from build123d import *

# Parameters (mm, degrees)
SKETCH1_W           = 77
SKETCH1_H           = 60
SKETCH1_W_2         = 71
SKETCH1_H_2         = 54
SKETCH1_R           = 1.75
BOSS_EXTRUDE1_DEPTH = 45
SKETCH2_R           = 1.75
CUT_EXTRUDE1_DEPTH  = 12
SKETCH3_W           = 77
SKETCH3_H           = 60
SKETCH3_R           = 1.75
BOSS_EXTRUDE2_DEPTH = 3
CUT_EXTRUDE2_DEPTH  = 10
SKETCH6_W           = 14
SKETCH6_H           = 9
CUT_EXTRUDE3_DEPTH  = 10
SKETCH7_R           = 1.1
CUT_EXTRUDE4_DEPTH  = 10
SKETCH9_W           = 60
SKETCH9_H           = 30
CUT_EXTRUDE5_DEPTH  = 169
SKETCH10_W          = 77
SKETCH10_H          = 60
BOSS_EXTRUDE3_DEPTH = 20
BOSS_EXTRUDE4_DEPTH = 1.5
SKETCH13_R          = 3
CUT_EXTRUDE6_DEPTH  = 1.5
FILLET1_R           = 1
BOSS_EXTRUDE5_DEPTH = 38
BOSS_EXTRUDE6_DEPTH = 38


with BuildPart() as part:
    # Sketch1 → Boss-Extrude1 (new body)
    with BuildSketch(Plane(origin=(0, 0, 0), x_dir=(1, 0, 0), z_dir=(0, 1, 0))):
        Rectangle(SKETCH1_W, SKETCH1_H)
        Rectangle(SKETCH1_W_2, SKETCH1_H_2, mode=Mode.SUBTRACT)
        with BuildLine():
            ThreePointArc((-25.5, -27), (-28.428932188, -19.928932188), (-35.5, -17))
            Line((-35.5, -17), (-35.5, -27))
            Line((-35.5, -27), (-25.5, -27))
        make_face()
        with Locations((-33, -23)):
            Circle(SKETCH1_R, mode=Mode.SUBTRACT)
        with BuildLine():
            Line((-25.5, 27), (-35.5, 27))
            Line((-35.5, 27), (-35.5, 17))
            ThreePointArc((-35.5, 17), (-28.428932188, 19.928932188), (-25.5, 27))
        make_face()
        with Locations((-33, 21)):
            Circle(SKETCH1_R, mode=Mode.SUBTRACT)
        with BuildLine():
            Line((35.5, 27), (25.5, 27))
            ThreePointArc((25.5, 27), (28.428932188, 19.928932188), (35.5, 17))
            Line((35.5, 17), (35.5, 27))
        make_face()
        with Locations((33, 21)):
            Circle(SKETCH1_R, mode=Mode.SUBTRACT)
        with BuildLine():
            Line((35.5, -27), (35.5, -17))
            ThreePointArc((35.5, -17), (28.428932188, -19.928932188), (25.5, -27))
            Line((25.5, -27), (35.5, -27))
        make_face()
        with Locations((33, -23)):
            Circle(SKETCH1_R, mode=Mode.SUBTRACT)
    extrude(amount=BOSS_EXTRUDE1_DEPTH)

    # Sketch2 → Cut-Extrude1 (cut)
    with BuildSketch(Plane(origin=(0, 45, 0), x_dir=(1, 0, 0), z_dir=(0, 1, 0))):
        with BuildLine():
            Line((-25.5, 27), (-35.5, 27))
            Line((-35.5, 27), (-35.5, 17))
            ThreePointArc((-35.5, 17), (-28.428932188, 19.928932188), (-25.5, 27))
        make_face()
        with Locations((-33, 21)):
            Circle(SKETCH2_R, mode=Mode.SUBTRACT)
        with BuildLine():
            Line((35.5, 17), (35.5, 27))
            Line((35.5, 27), (25.5, 27))
            ThreePointArc((25.5, 27), (28.428932188, 19.928932188), (35.5, 17))
        make_face()
        with Locations((33, 21)):
            Circle(SKETCH2_R, mode=Mode.SUBTRACT)
        with BuildLine():
            Line((-25.5, -27), (-35.5, -27))
            Line((-35.5, -27), (-35.5, -17))
            ThreePointArc((-35.5, -17), (-28.428932188, -19.928932188), (-25.5, -27))
        make_face()
        with Locations((-33, -23)):
            Circle(SKETCH2_R, mode=Mode.SUBTRACT)
        with BuildLine():
            Line((25.5, -27), (35.5, -27))
            Line((35.5, -27), (35.5, -17))
            ThreePointArc((35.5, -17), (28.428932188, -19.928932188), (25.5, -27))
        make_face()
        with Locations((33, -23)):
            Circle(SKETCH2_R, mode=Mode.SUBTRACT)
    extrude(amount=-CUT_EXTRUDE1_DEPTH, mode=Mode.SUBTRACT)

    # Sketch3 → Boss-Extrude2 (add)
    with BuildSketch(Plane.XZ):
        Rectangle(SKETCH3_W, SKETCH3_H)
        with Locations((33, -21)):
            Circle(SKETCH3_R, mode=Mode.SUBTRACT)
        with Locations((-33, -21)):
            Circle(SKETCH3_R, mode=Mode.SUBTRACT)
        with Locations((33, 23)):
            Circle(SKETCH3_R, mode=Mode.SUBTRACT)
        with Locations((-33, 23)):
            Circle(SKETCH3_R, mode=Mode.SUBTRACT)
    extrude(amount=-BOSS_EXTRUDE2_DEPTH)

    # Sketch4 → Cut-Extrude2 (cut)
    with BuildSketch(Plane(origin=(0, 0, -30), x_dir=(-1, 0, 0), z_dir=(0, 0, -1))):
        with BuildLine():
            Line((-18.5, 43), (-10.5, 43))
            ThreePointArc((-10.5, 43), (-9.792893219, 42.707106781), (-9.5, 42))
            Line((-9.5, 42), (-9.5, 39))
            ThreePointArc((-9.5, 39), (-9.792893219, 38.292893219), (-10.5, 38))
            Line((-10.5, 38), (-18.5, 38))
            ThreePointArc((-18.5, 38), (-19.207106781, 38.292893219), (-19.5, 39))
            Line((-19.5, 39), (-19.5, 42))
            ThreePointArc((-19.5, 42), (-19.207106781, 42.707106781), (-18.5, 43))
        make_face()
    extrude(amount=-CUT_EXTRUDE2_DEPTH, mode=Mode.SUBTRACT)

    # Sketch6 → Cut-Extrude3 (cut)
    with BuildSketch(Plane.ZY.offset(38.5)):
        with Locations((10, 38)):
            Rectangle(SKETCH6_W, SKETCH6_H)
    extrude(amount=-CUT_EXTRUDE3_DEPTH, mode=Mode.SUBTRACT)

    # Sketch7 → Cut-Extrude4 (cut)
    with BuildSketch(Plane(origin=(0, 45, 0), x_dir=(1, 0, 0), z_dir=(0, 1, 0))):
        with Locations((-37, 28.5)):
            Circle(SKETCH7_R)
        with Locations((37, 28.5)):
            Circle(SKETCH7_R)
        with Locations((37, -28.5)):
            Circle(SKETCH7_R)
        with Locations((-37, -28.5)):
            Circle(SKETCH7_R)
    extrude(amount=-CUT_EXTRUDE4_DEPTH, mode=Mode.SUBTRACT)

    # Sketch9 → Cut-Extrude5 (cut)
    with BuildSketch(Plane.ZY.offset(38.5)):
        with Locations((0, 15)):
            Rectangle(SKETCH9_W, SKETCH9_H)
    extrude(amount=-CUT_EXTRUDE5_DEPTH, mode=Mode.SUBTRACT)

    # Sketch10 → Boss-Extrude3 (add)
    with BuildSketch(Plane.XZ.offset(-30)):
        Rectangle(SKETCH10_W, SKETCH10_H)
        Polygon((-35.5, 17), (-35.5, 27), (-25.5, 27), (25.5, 27), (35.5, 27), (35.5, 17), (35.5, -17), (35.5, -27), (25.5, -27), (-25.5, -27), (-35.5, -27), (-35.5, -17), align=None, mode=Mode.SUBTRACT)
    extrude(amount=BOSS_EXTRUDE3_DEPTH)

    # Sketch11 → Boss-Extrude4 (add)
    with BuildSketch(Plane.XZ.offset(-30)):
        with BuildLine():
            Line((35.5, 17), (35.5, -17))
            ThreePointArc((35.5, -17), (28.428932188, -19.928932188), (25.5, -27))
            Line((25.5, -27), (-25.5, -27))
            ThreePointArc((-25.5, -27), (-28.428932188, -19.928932188), (-35.5, -17))
            Line((-35.5, -17), (-35.5, 17))
            ThreePointArc((-35.5, 17), (-28.428932188, 19.928932188), (-25.5, 27))
            Line((-25.5, 27), (25.5, 27))
            ThreePointArc((25.5, 27), (28.428932188, 19.928932188), (35.5, 17))
        make_face()
    extrude(amount=-BOSS_EXTRUDE4_DEPTH)

    # Sketch13 → Cut-Extrude6 (cut)
    with BuildSketch(Plane.XZ.offset(-30)):
        with Locations((22.535934278, 21.73153163)):
            Circle(SKETCH13_R)
    extrude(amount=-CUT_EXTRUDE6_DEPTH, mode=Mode.SUBTRACT)

    # Fillet1
    fillet1_edges = [part.edges().sort_by_distance(p)[0] for p in [
        (38.5, 27.5, 30),
        (-38.5, 27.5, 30),
        (-38.5, 27.5, -30),
        (38.5, 27.5, -30),
    ]]
    fillet(fillet1_edges, radius=FILLET1_R)

    # Sketch14 → Boss-Extrude5 (add)
    with BuildSketch(Plane(origin=(0, 45, 0), x_dir=(1, 0, 0), z_dir=(0, 1, 0))):
        with BuildLine():
            Line((-38.5, 29), (-38.5, 25.901923789))
            ThreePointArc((-38.5, 25.901923789), (-39.121320344, 30.621320344), (-34.401923789, 30))
            Line((-34.401923789, 30), (-37.5, 30))
            ThreePointArc((-37.5, 30), (-38.207106781, 29.707106781), (-38.5, 29))
        make_face()
    extrude(amount=-BOSS_EXTRUDE5_DEPTH)

    # Sketch15 → Boss-Extrude6 (add)
    with BuildSketch(Plane(origin=(0, 45, 0), x_dir=(1, 0, 0), z_dir=(0, 1, 0))):
        with BuildLine():
            Line((38.5, 29), (38.5, 25.901923789))
            ThreePointArc((38.5, 25.901923789), (39.121320344, 30.621320344), (34.401923789, 30))
            Line((34.401923789, 30), (37.5, 30))
            ThreePointArc((37.5, 30), (38.207106781, 29.707106781), (38.5, 29))
        make_face()
        with BuildLine():
            Line((37.5, -30), (34.401923789, -30))
            ThreePointArc((34.401923789, -30), (39.121320344, -30.621320344), (38.5, -25.901923789))
            Line((38.5, -25.901923789), (38.5, -29))
            ThreePointArc((38.5, -29), (38.207106781, -29.707106781), (37.5, -30))
        make_face()
        with BuildLine():
            ThreePointArc((-38.5, -25.901923789), (-39.121320344, -30.621320344), (-34.401923789, -30))
            Line((-34.401923789, -30), (-37.5, -30))
            ThreePointArc((-37.5, -30), (-38.207106781, -29.707106781), (-38.5, -29))
            Line((-38.5, -29), (-38.5, -25.901923789))
        make_face()
    extrude(amount=-BOSS_EXTRUDE6_DEPTH)


solid = part.part
Design review of the part built by this model. Coordinates are the model's own, in mm. A direction names the side the tool comes from. Coordinates: 2 decimals unless noted, no trailing zeros. Order: outer loops, then holes, each group sorted by start corner. A loop starts at its lowest first (then second) coordinate and runs counter-clockwise, first axis right, second up. Notation, with made-up numbers: (-24.75, 9.25) -> (30.25, 9.25) arc R17 ccw to (30.25, 38.25) -> close; hole circle Ø7 at (67, 43.5). An arc over 180 degrees is marked (long way). One line per item, written item: value.
1) Machinability: for faces 3 (the face through (19.5, 40, -29)), 4 (the face through (-39.175, 26.266, -30.566)), 5 (the face through (-31, 33, -23)), 6 (the face through (36, 9, -30)), which of the approach directions +Z, -Z, +X, -X, +Y, -Y give a long, thin tool a straight path to every point of the face, cutting with its end or side? Answer none if there is none.
Output values:
face 3: -Z
face 4: +Y, -Y
face 5: +Y
face 6: -Y
2) Clearance check with flat-ended pins moving along their axes: P1, Ø11, axis at x = -1.5, y = 35.5, coming from the +Z side; P2, Ø2, axis at x = -33, z = -21, coming from the -Y side; P3, Ø4, axis at y = 27.5, z = 0.5, coming from the -X side; P4, Ø3, axis at x = -17, y = 18.5, coming from the -Z side. State where each tip first meets the part, or that it passes through.
Output values:
P1: stops at z = 30
P2: passes through
P3: stops at x = -38.5
P4: stops at z = -30
3) We need section A-A, the plane x = 12. Give the boundary of the cut face in (y, z), then the cut area to 3 significant figures.
Output values:
outline: (10, -30) -> (38, -30) -> (38, -27) -> (31.5, -27) -> (31.5, 27) -> (45, 27) -> (45, 30) -> (10, 30) -> (10, 27) -> (30, 27) -> (30, -27) -> (10, -27) -> close; (43, -30) -> (45, -30) -> (45, -27) -> (43, -27) -> close
area: 276 mm2
4) We need section C-C, the plane z = -9.5. Give the boundary of the cut face in (x, y).
Output values:
outline: (-38.5, 10) -> (-35.5, 10) -> (-35.5, 30) -> (35.5, 30) -> (35.5, 10) -> (38.5, 10) -> (38.5, 45) -> (35.5, 45) -> (35.5, 31.5) -> (-35.5, 31.5) -> (-35.5, 45) -> (-38.5, 45) -> close
5) We need section B-B, the plane y = 11. Give the boundary of the cut face in (x, z), then the cut area to 3 significant figures.
Output values:
outline: (-38.5, -25.9) arc R3 ccw (long way) to (-34.4, -30) -> (34.4, -30) arc R3 ccw (long way) to (38.5, -25.9) -> (38.5, 25.9) arc R3 ccw (long way) to (34.4, 30) -> (-34.4, 30) arc R3 ccw (long way) to (-38.5, 25.9) -> close; hole (-35.5, -27) -> (35.5, -27) -> (35.5, 27) -> (-35.5, 27) -> close
area: 827 mm2
6) Draft analysis for pull direction X (two halves, no side actions). For faces 1 (the face through (0, 45, -28)), 2 (the face through (-34.29, 31.48, -22.18)), state which applies: +X half, -X half, draft (parallel to the pull), parting line (faces both ways), or undercut.
Output values:
face 1: draft
face 2: undercut
7) We need section D-D, the plane x = -23. Give the boundary of the cut face in (y, z).
Output values:
outline: (10, -30) -> (45, -30) -> (45, -27) -> (31.5, -27) -> (31.5, 27) -> (45, 27) -> (45, 30) -> (10, 30) -> (10, 27) -> (30, 27) -> (30, -27) -> (10, -27) -> close
8) To check wall thickness, follow probe 1 along Z at (x, y) = (37, 42.75); probe 2 along Z at (x, y) = (33, 30.95); probe 3 along Z at (x, y) = (-15, 15.5). State the ranges of each line that lie inside material, in increasing order. Write a range as [from, to].
Output values:
probe 1: z = [-31.5, -29.6], [-27.4, 27.4], [29.6, 31.5]
probe 2: z = [-30, -22.75], [-19.25, 21.25], [24.75, 30]
probe 3: z = [-30, -27], [27, 30]
